Here's how the part is built. I have some questions about the finished solid (model axes, mm). A direction names the side the tool comes from. Coordinates: 2 decimals unless noted, no trailing zeros. Write each loop counter-clockwise with the first axis right and the second up, starting at its lowest first coordinate (ties: lowest second). Pieces come first, ordered by that corner, then holes. Notation, with made-up numbers: (-1.5, 7) -> (3.5, 7) arc R14 ccw to (3.5, 31) -> close; hole circle Ø9 at (3.25, 69.25). An arc over 180 degrees is marked (long way). Put each result on its own line as item: value.
```python
from build123d import *

# Parameters (mm, degrees)
SKETCH1_W           = 33
SKETCH1_H           = 28
BOSS_EXTRUDE1_DEPTH = 46
SKETCH2_W           = 17.5
SKETCH2_H           = 41
CUT_EXTRUDE1_DEPTH  = 59.318093247
EXTRUDE_S_DEPTH     = 3
BOSS_EXTRUDE3_DEPTH = 27
FILLET1_START       = -3.5
FILLET1_DEPTH       = 5.287760197
FILLET1_START_2     = -13.5
FILLET1_2_DEPTH     = 27
FILLET2_R           = 16.5
FILLET3_R           = 6
SKETCH5_W           = 13
SKETCH5_H           = 23
CUT_EXTRUDE3_DEPTH  = 9
SKETCH6_R           = 6.5
CUT_EXTRUDE4_DEPTH  = 9
SKETCH7_R           = 1
CUT_EXTRUDE5_DEPTH  = 8
SKETCH8_R           = 1.3
SKETCH8_R_2         = 2.5
CUT_EXTRUDE6_DEPTH  = 47.360004895


with BuildPart() as part:
    # Sketch1 → Boss-Extrude1 (new body)
    with BuildSketch(Plane(origin=(0, 0, 0), x_dir=(1, 0, 0), z_dir=(0, 1, 0))):
        Rectangle(SKETCH1_W, SKETCH1_H)
    extrude(amount=BOSS_EXTRUDE1_DEPTH)

    # Sketch2 → Cut-Extrude1 (cut, through all)
    with BuildSketch(Plane(origin=(16.5, 0, 0), x_dir=(0, 0, -1), z_dir=(1, 0, 0))):
        with Locations((-5.25, 25.5)):
            Rectangle(SKETCH2_W, SKETCH2_H)
    extrude(amount=-CUT_EXTRUDE1_DEPTH, mode=Mode.SUBTRACT)

    # Sketch3 → Extrude S (add)
    with BuildSketch(Plane(origin=(16.5, 0, 0), x_dir=(0, 0, -1), z_dir=(1, 0, 0))):
        with BuildLine():
            Line((-14, 5), (3.5, 5))
            Line((3.5, 5), (3.5, 46))
            Line((3.5, 46), (2, 46))
            add(Edge.make_bspline(
                [(2, 46), (-1.17854194, 23.414715012), (-14, 5)],
                knots=[0, 0, 0, 1, 1, 1], degree=2))
        make_face()
    extrude_s = extrude(amount=-EXTRUDE_S_DEPTH)

    # Mirror1: Extrude S across plane
    add(extrude_s.mirror(Plane(origin=(0, 0, 0), x_dir=(0, 0, 1), z_dir=(1, 0, 0))))

    # Sketch4 → Boss-Extrude3 (add)
    with BuildSketch(Plane.ZY.offset(-13.5)):
        with BuildLine():
            Line((-3.5, 46), (-3.5, 43))
            Line((-3.5, 43), (-1.532109396, 43))
            add(Edge.make_bspline(
                [(-1.532109396, 43), (-1.787586761, 44.490687359), (-1.999999999, 45.999999992)],
                knots=[0.933172744, 0.933172744, 0.933172744, 1, 1, 1], degree=2))
            Line((-1.999999999, 45.999999992), (-3.5, 46))
        make_face()
    extrude(amount=BOSS_EXTRUDE3_DEPTH)

    # Fillet1: read off the stored shape, not the designer's step
    # Fillet1 outline → Fillet1 (add)
    with BuildSketch(Plane.XY.offset(FILLET1_START)):
        with BuildLine():
            Line((-13.5, 43), (-13.5, 29.5))
            ThreePointArc((-13.5, 29.5), (-9.545941546, 39.045941546), (0, 43))
            Line((0, 43), (-13.5, 43))
        make_face()
        with BuildLine():
            Line((13.5, 43), (0, 43))
            ThreePointArc((0, 43), (9.545941546, 39.045941546), (13.5, 29.5))
            Line((13.5, 29.5), (13.5, 43))
        make_face()
    extrude(amount=FILLET1_DEPTH)

    # Fillet1 2 outline → Fillet1 2 (cut)
    with BuildSketch(Plane.YZ.offset(FILLET1_START_2)):
        with BuildLine():
            add(Edge.make_bspline(
                [(43, -1.532109396), (36.047422478, -0.340560963), (29.499999971, 1.787760107)],
                knots=[0.066827257, 0.066827257, 0.066827257, 0.378510105, 0.378510105, 0.378510105], degree=2))
            Line((43, -1.532109396), (43, 1.787760197))
            Line((43, 1.787760197), (29.499999971, 1.787760107))
        make_face()
    extrude(amount=FILLET1_2_DEPTH, mode=Mode.SUBTRACT)

    # Fillet2
    # the kernel refuses this fillet: 16.5 mm, written as the material it takes off along each edge
    with BuildSketch(Plane(origin=(16.5, 46, -55.25), x_dir=(0, -1, 0), z_dir=(0, 0, 1)), Plane(origin=(-16.5, 46, 39.25), x_dir=(0, -1, 0), z_dir=(0, 0, -1))) as fillet2_piece_1:
        with BuildLine():
            CenterArc((FILLET2_R, -FILLET2_R), FILLET2_R, 90, 90)
            Line((0, -FILLET2_R), (0, 0))
            Line((0, 0), (FILLET2_R, 0))
        make_face()
    extrude(amount=94.5, mode=Mode.SUBTRACT)

    # Fillet3
    # the kernel refuses this fillet: 6 mm, written as the material it takes off along each edge
    with BuildSketch(Plane(origin=(16.5, -15, 14), x_dir=(0, 0, -1), z_dir=(0, 1, 0)), Plane(origin=(-16.5, -15, 14), x_dir=(1, 0, 0), z_dir=(0, 1, 0))) as fillet3_piece_1:
        with BuildLine():
            CenterArc((FILLET3_R, FILLET3_R), FILLET3_R, 180, 90)
            Line((0, FILLET3_R), (0, 0))
            Line((0, 0), (FILLET3_R, 0))
        make_face()
    extrude(amount=35, mode=Mode.SUBTRACT)

    # Sketch5 → Cut-Extrude3 (cut)
    with BuildSketch(Plane.XY.offset(-3.5)):
        with Locations((0, 23)):
            Rectangle(SKETCH5_W, SKETCH5_H)
    extrude(amount=-CUT_EXTRUDE3_DEPTH, mode=Mode.SUBTRACT)

    # Sketch6 → Cut-Extrude4 (cut)
    with BuildSketch(Plane.XY.offset(-12.5)):
        with Locations((0, 28)):
            Circle(SKETCH6_R)
    extrude(amount=-CUT_EXTRUDE4_DEPTH, mode=Mode.SUBTRACT)

    # Sketch7 → Cut-Extrude5 (cut)
    with BuildSketch(Plane.XY.offset(-3.5)):
        with Locations((0, 36.8)):
            Circle(SKETCH7_R)
        with Locations((0, 9.2)):
            Circle(SKETCH7_R)
    extrude(amount=-CUT_EXTRUDE5_DEPTH, mode=Mode.SUBTRACT)

    # Sketch8 → Cut-Extrude6 (cut, through all)
    with BuildSketch(Plane(origin=(0, 5, 0), x_dir=(1, 0, 0), z_dir=(0, 1, 0))):
        with Locations(Location((-0.5, 0, 0), (0, 0, 270))):
            Circle(SKETCH8_R)
        with Locations(Location((-5, 0, 0), (0, 0, 270))):
            Circle(SKETCH8_R_2)
        with Locations(Location((-9.5, 0, 0), (0, 0, 270))):
            Circle(SKETCH8_R)
    extrude(amount=-CUT_EXTRUDE6_DEPTH, mode=Mode.SUBTRACT)


solid = part.part
```
Item 1: Imagine slicing it at A-A on z = -9. Write out the boundary of the cut face in (x, y), then the cut area to 3 significant figures.
Output:
outline: (-16.5, 0) -> (16.5, 0) -> (16.5, 29.5) arc R16.5 ccw to (-16.5, 29.5) -> close; hole (-6.5, 11.5) -> (6.5, 11.5) -> (6.5, 34.5) -> (-6.5, 34.5) -> close; hole circle Ø2 at (0, 9.2); hole circle Ø2 at (0, 36.8)
area: 1,100 mm²
Item 2: Which directions (+Z, -Z, +X, -X, +Y, -Y) give clear straight access to the entire face, cutting with the end or side of a thin tool? Please do faces 5 (the flat face through (16.5, 15, -3)), 6 (the cylindrical face through (-8.21, 2.54, -0.17)), 7 (the flat face through (13.5, 15, 3)).
Output:
face 5: +Z, -Z, +X, +Y, -Y
face 6: -Y
face 7: +Z
Item 3: Imagine slicing it at B-B on x = -5. State how many separate pieces and enclosed holes the cut face has, then the cut area to 3 significant figures.
Output:
separate pieces: 3
enclosed holes: 0
area: 324 mm²
Item 4: For P1, Ø1.6, axis at x = 0, y = 9.2, coming from the +Z side; P2, Ø3, axis at x = -11.5, z = 9.5, coming from the +Y side; P3, Ø6, axis at x = -5, y = 30, coming from the +Z side, each with a flat end and sliding along its axis, tell me the tip position at first contact or that it passes through.
Output:
P1: stops at z = -11.5
P2: stops at y = 5
P3: stops at z = -3.5
Item 5: Please list where these lines run through material, in increasing order: line 1 along Y through (x, z) = (0, -8.75); line 2 along X through (y, z) = (12.5, 5.5); line 3 along X through (y, z) = (28, -13.6). Write a range as from..to.
Output:
line 1: y = 0..8.2, 10.2..11.5, 34.5..35.8, 37.8..46
line 2: x = -16.5..-13.5, 13.5..16.5
line 3: x = -16.5..-6.5, 6.5..16.5
Item 6: If we mould it in two halves opening along X, with no side actions, what happens to faces 1 (the flat face through (0, 5, 5)), 2 (the flat face through (0, 2, 14)), 3 (the cylindrical face through (15.377, 4.015, 11.495)), 4 (the flat face through (-13.5, 15, 3))? For each: released by +X, released by -X, zero draft, split by the parting line, or undercut.
Output:
face 1: undercut
face 2: zero draft
face 3: released by +X
face 4: undercut
